The listing builds one solid part. Answer for the finished solid, in the listing's coordinates (mm). A direction names the side the tool comes from. Give positions to 0.01 mm unless a question says otherwise; leave off trailing zeros. Write each loop counter-clockwise with the first axis right and the second up, starting at its lowest first coordinate (ties: lowest second). Pieces come first, ordered by that corner, then holes. Notation, with made-up numbers: (74, -25) - (120, -25) arc R21 ccw to (120, 13) - close; hole circle Ø9 at (5.25, -35). An arc over 180 degrees is marked (long way). Use a Markdown table: item, result. Add a question column.
from build123d import *

# Parameters (mm, degrees)
BOSS_EXTRUDE1_DEPTH = 20
CUT_EXTRUDE1_DEPTH  = 10
CUT_EXTRUDE2_DEPTH  = 10
BOSS_EXTRUDE2_DEPTH = 2


with BuildPart() as part:
    # Sketch2 → Boss-Extrude1 (new body)
    with BuildSketch(Plane.XY):
        Polygon((0, 0), (0, 28), (3, 28), (3, 3), (28, 3), (28, 0), align=None)
    extrude(amount=-BOSS_EXTRUDE1_DEPTH)

    # Sketch4 → Cut-Extrude1 (cut)
    with BuildSketch(Plane(origin=(0, 3, 0), x_dir=(1, 0, 0), z_dir=(0, 1, 0))):
        with BuildLine():
            Line((9.8, 12.95), (21.2, 12.95))
            ThreePointArc((21.2, 12.95), (24.15, 10), (21.2, 7.05))
            Line((21.2, 7.05), (9.8, 7.05))
            ThreePointArc((9.8, 7.05), (6.85, 10), (9.8, 12.95))
        make_face()
    extrude(amount=-CUT_EXTRUDE1_DEPTH, mode=Mode.SUBTRACT)

    # Sketch5 → Cut-Extrude2 (cut)
    with BuildSketch(Plane(origin=(3, 0, 0), x_dir=(0, 0, -1), z_dir=(1, 0, 0))):
        with BuildLine():
            Line((12.95, 21.2), (12.95, 9.8))
            ThreePointArc((12.95, 9.8), (10, 6.85), (7.05, 9.8))
            Line((7.05, 9.8), (7.05, 21.2))
            ThreePointArc((7.05, 21.2), (10, 24.15), (12.95, 21.2))
        make_face()
    extrude(amount=-CUT_EXTRUDE2_DEPTH, mode=Mode.SUBTRACT)

    # Sketch6 → Boss-Extrude2 (add)
    with BuildSketch(Plane.XY):
        Polygon((3, 28), (5, 28), (5, 25), (25, 5), (28, 5), (28, 3), (3, 3), align=None)
    boss_extrude2 = extrude(amount=-BOSS_EXTRUDE2_DEPTH)

    # Mirror4: Boss-Extrude2 across plane
    add(boss_extrude2.mirror(Plane(origin=(0, 0, -10), x_dir=(1, 0, 0), z_dir=(0, 0, -1))))


solid = part.part
1. The part is cut by section A-A (z = -10). Give the vertices of the cut face in (x, y).
2. The part is cut by section C-C (x = 12.5). Give the vertices of the cut face in (y, z), and give its area (3 significant figures).
3. Which of the six approach directions +Z, -Z, +X, -X, +Y, -Y give full straight-line access (tool end or side, diameter ignored) to faces 5 (the flat face through (5, 27, -19)), 6 (the flat face through (14, 0, -5)), 7 (the cylindrical face through (1.52, 24.15, -9.94)), 8 (the flat face through (15, 2, -12.95)), 9 (the flat face through (3, 15.7, -13.4))?
4. Consider L1, parallel to Z at x = 13.75, y = 1.5; L2, parallel to X at y = 12, z = -3; L3, parallel to Z at x = 18.5, y = 5.5. Determine where each line is inside the solid, lowest interval first. Write a range as [from, to].
5. The part is cut by section B-B (y = 19.5). Give the vertices of the cut face in (x, z).
6. Given P1, Ø0.6, axis at y = 26.5, z = -1, coming from the +X side; P2, Ø1.5, axis at y = 12, z = -10.5, coming from the +X side; P3, Ø5, axis at y = 16.5, z = -11, coming from the +X side; P4, Ø2, axis at x = 26.5, z = -19.5, coming from the +Y side, each flat-ended and moving along its own axis, determine where each tip first touches the part or whether it passes through.
7. For a pull along Z with two mould halves and no side action, classify faces 1 (the flat face through (15.3, 3, -13.4)), 2 (the cylindrical face through (1.52, 6.85, -10.06)), 3 (the flat face through (15, 15, -1)), 4 (the flat face through (11, 11, -20)) as released by +Z, released by -Z, zero draft, split by the parting line, or undercut.
8. The part is cut by section D-D (z = -14.75). Give the vertices of the cut face in (x, y), and give its area (3 significant figures).
Check values:
| question | item | result |
|---|---|---|
| 1 | outline | (0, 0) - (6.85, 0) - (6.85, 3) - (3, 3) - (3, 6.85) - (0, 6.85) - close; (0, 24.15) - (3, 24.15) - (3, 28) - (0, 28) - close; (24.15, 0) - (28, 0) - (28, 3) - (24.15, 3) - close |
| 2 | outline | (0, -20) - (17.5, -20) - (17.5, -18) - (3, -18) - (3, -12.95) - (0, -12.95) - close; (0, -7.05) - (3, -7.05) - (3, -2) - (17.5, -2) - (17.5, 0) - (0, 0) - close |
| 2 | area | 100 mm2 |
| 3 | face 5 | +Z, -Z, +X, +Y |
| 3 | face 6 | +Z, -Z, +X, -X, -Y |
| 3 | face 7 | +X, -X |
| 3 | face 8 | +Y, -Y |
| 3 | face 9 | +X, +Y |
| 4 | L1 | z = [-20, -12.95], [-7.05, 0] |
| 4 | L2 | x = [0, 3] |
| 4 | L3 | z = [-20, -18], [-2, 0] |
| 5 | outline | (0, -20) - (10.5, -20) - (10.5, -18) - (3, -18) - (3, -12.95) - (0, -12.95) - close; (0, -7.05) - (3, -7.05) - (3, -2) - (10.5, -2) - (10.5, 0) - (0, 0) - close |
| 6 | P1 | stops at x = 5 |
| 6 | P2 | passes through |
| 6 | P3 | stops at x = 3 |
| 6 | P4 | stops at y = 5 |
| 7 | face 1 | undercut |
| 7 | face 2 | undercut |
| 7 | face 3 | zero draft |
| 7 | face 4 | released by -Z |
| 8 | outline | (0, 0) - (28, 0) - (28, 3) - (3, 3) - (3, 28) - (0, 28) - close |
| 8 | area | 159 mm2 |
